Design review of the part built by this model. Coordinates are the model's own, in mm. Face numbers are marked on the shaded views. A direction names the side the tool comes from. Give positions to 0.01 mm unless a question says otherwise; leave off trailing zeros. Write each loop counter-clockwise with the first axis right and the second up, starting at its lowest first coordinate (ties: lowest second). Pieces come first, ordered by that corner, then holes. Notation, with made-up numbers: M 5.5,58.25 L 37.5,58.25 A16 cw 37.5,73.25 Z; hole C 22.25,87 d3. An arc over 180 degrees is marked long. Use a Markdown table: item, result. Add a question column.
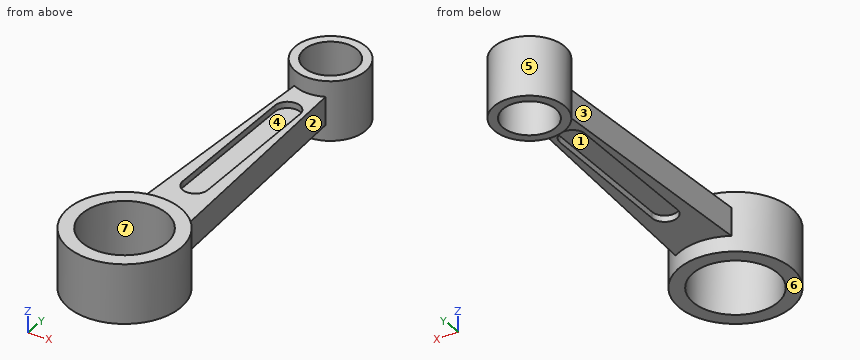
```python
from build123d import *

# Parameters (mm, degrees)
SKETCH1_R             = 22.5
SKETCH1_R_2           = 16.9
BOSS_EXTRUDE1_DEPTH   = 19
SKETCH1_R_3           = 36
SKETCH1_R_4           = 27
BOSS_EXTRUDE1_2_DEPTH = 19
BOSS_EXTRUDE2_DEPTH   = 9
CUT_EXTRUDE1_DEPTH    = 4


with BuildPart() as part:
    # Sketch1 → Boss-Extrude1 (new, symmetric)
    with BuildSketch(Plane.XY):
        Circle(SKETCH1_R)
        Circle(SKETCH1_R_2, mode=Mode.SUBTRACT)
    extrude(amount=BOSS_EXTRUDE1_DEPTH, both=True)



with BuildPart() as body_2:
    # Sketch1 → Boss-Extrude1 2 (new, symmetric)
    with BuildSketch(Plane.XY):
        with Locations((0, -201.2)):
            Circle(SKETCH1_R_3)
        with Locations((0, -201.2)):
            Circle(SKETCH1_R_4, mode=Mode.SUBTRACT)
    extrude(amount=BOSS_EXTRUDE1_2_DEPTH, both=True)


with BuildPart() as part_1:
    add(part.part)

    add(body_2.part)  # Boss-Extrude2 merges body 2
    # Sketch1_3 → Boss-Extrude2 (add, symmetric)
    with BuildSketch(Plane.XY):
        with BuildLine():
            Line((0, -165.2), (0, -22.5))
            ThreePointArc((0, -22.5), (-5.135562367, -21.906072199), (-10, -20.155644371))
            Line((-10, -20.155644371), (-17.849697213, -169.936789841))
            ThreePointArc((-17.849697213, -169.936789841), (-9.233754228, -166.404342471), (0, -165.2))
        make_face()
        with BuildLine():
            ThreePointArc((10, -20.155644371), (5.135562367, -21.906072199), (0, -22.5))
            Line((0, -22.5), (0, -165.2))
            ThreePointArc((0, -165.2), (9.233754228, -166.404342471), (17.849697213, -169.936789841))
            Line((17.849697213, -169.936789841), (10, -20.155644371))
        make_face()
    extrude(amount=BOSS_EXTRUDE2_DEPTH, both=True)

    # Sketch2 → Cut-Extrude1 (cut)
    with BuildSketch(Plane.XY.offset(9)):
        with BuildLine():
            Line((-8, -132.1), (-8, -42.1))
            ThreePointArc((-8, -42.1), (0, -34.1), (8, -42.1))
            Line((8, -42.1), (8, -132.1))
            ThreePointArc((8, -132.1), (0, -140.1), (-8, -132.1))
        make_face()
    cut_extrude1 = extrude(amount=-CUT_EXTRUDE1_DEPTH, mode=Mode.SUBTRACT)

    # Mirror1: Cut-Extrude1 across plane
    add(cut_extrude1.mirror(Plane.XY), mode=Mode.SUBTRACT)


solid = part_1.part
```
(1) The part is to be moulded in two halves that separate along X. For the marked faces 5, 6 and 7, say which applies: released by +X, released by -X, zero draft, split by the parting line, or undercut.
(2) Wall thickness on L1, parallel to Y at x = 0, z = -6; L2, parallel to Y at x = 0, z = -10; L3, parallel to Y at x = 0, z = 4: over which ranges is each line inside the solid? List them lowest first.
(3) Add section A-A on y = 0. Give the boundary of the cut face in (x, z).
(4) Machinability: for the marked faces 1, 2, 3 and 4, which of the approach directions +Z, -Z, +X, -X, +Y, -Y give a long, thin tool a straight path to every point of the face, cutting with its end or side? Answer none if there is none.
(5) Add section B-B on z = -16. Give the boundary of the cut face in (x, y), then the cut area to 3 significant figures.
(6) Add section C-C on x = -4.5. Give the boundary of the cut face in (y, z).
(7) Add section D-D on z = 2. Give the boundary of the cut face in (x, y).
(8) For pin 1 (1.2 mm diameter, centred on y = -75.5, z = 7.5, fed in from +X); pin 2 (4.5 mm diameter, centred on y = -75.5, z = 6, fed in from -X); pin 3 (6 mm diameter, centred on x = -28.5, z = 10.5, fed in from +Y), all flat-tipped, find the tip position at first contact; note any pin that passes through.
From the geometry:
| question | item | result |
|---|---|---|
| 1 | face 5 | split by the parting line |
| 1 | face 6 | zero draft |
| 1 | face 7 | undercut |
| 2 | L1 | y = -237.2 to -228.2, -174.2 to -140.1, -34.1 to -16.9, 16.9 to 22.5 |
| 2 | L2 | y = -237.2 to -228.2, -174.2 to -165.2, -22.5 to -16.9, 16.9 to 22.5 |
| 2 | L3 | y = -237.2 to -228.2, -174.2 to -16.9, 16.9 to 22.5 |
| 3 | outline | M -22.5,-19 L -16.9,-19 L -16.9,19 L -22.5,19 Z; M 16.9,-19 L 22.5,-19 L 22.5,19 L 16.9,19 Z |
| 4 | face 1 | -Z |
| 4 | face 2 | +Z, -Z, +X |
| 4 | face 3 | +Z, -Z, -X |
| 4 | face 4 | +Z |
| 5 | outline | C 0,-201.2 d72; C 0,0 d45; hole C 0,-201.2 d54; hole C 0,0 d33.8 |
| 5 | area | 2,470 mm^2 |
| 6 | outline | M -236.92,-19 L -227.82,-19 L -227.82,19 L -236.92,19 Z; M -174.58,-19 L -165.48,-19 L -165.48,-9 L -138.71,-9 L -138.71,-5 L -35.49,-5 L -35.49,-9 L -22.05,-9 L -22.05,-19 L -16.29,-19 L -16.29,19 L -22.05,19 L -22.05,9 L -35.49,9 L -35.49,5 L -138.71,5 L -138.71,9 L -165.48,9 L -165.48,19 L -174.58,19 Z; M 16.29,-19 L 22.05,-19 L 22.05,19 L 16.29,19 Z |
| 7 | outline | M -17.85,-169.94 A36 ccw long 17.85,-169.94 L 10,-20.16 A22.5 ccw long -10,-20.16 Z; hole C 0,-201.2 d54; hole C 0,0 d33.8 |
| 8 | pin 1 | stops at x = 12.93 |
| 8 | pin 2 | stops at x = -13.02 |
| 8 | pin 3 | stops at y = -175.79 |
